```python
from build123d import *

# Parameters (mm, degrees)
AUFSATZ_LINEAR_AUSTRAGEN1_DEPTH = 380


with BuildPart() as part:
    # Skizze1 → Aufsatz-Linear austragen1 (new body)
    with BuildSketch(Plane.XY):
        with BuildLine():
            Line((9.896623228, -8.686160957), (9.896623228, -3.686160957))
            Line((9.896623228, -3.686160957), (9.396623228, -3.686160957))
            Line((9.396623228, -3.686160957), (9.396623228, -3.186160957))
            Line((9.396623228, -3.186160957), (8.396623228, -3.186160957))
            Line((8.396623228, -3.186160957), (8.396623228, -6.186160957))
            Line((8.396623228, -6.186160957), (6.957283398, -6.186160957))
            Line((6.957283398, -6.186160957), (4.396623228, -3.625500787))
            Line((4.396623228, -3.625500787), (4.396623228, 3.253178873))
            Line((4.396623228, 3.253178873), (6.957283398, 5.813839043))
            Line((6.957283398, 5.813839043), (8.396623228, 5.813839043))
            Line((8.396623228, 5.813839043), (8.396623228, 2.813839043))
            Line((8.396623228, 2.813839043), (9.396623228, 2.813839043))
            Line((9.396623228, 2.813839043), (9.396623228, 3.313839043))
            Line((9.396623228, 3.313839043), (9.896623228, 3.313839043))
            Line((9.896623228, 3.313839043), (9.896623228, 8.313839043))
            ThreePointArc((9.896623228, 8.313839043), (9.457283398, 9.374499213), (8.396623228, 9.813839043))
            Line((8.396623228, 9.813839043), (3.396623228, 9.813839043))
            Line((3.396623228, 9.813839043), (3.396623228, 9.313839043))
            Line((3.396623228, 9.313839043), (2.896623228, 9.313839043))
            Line((2.896623228, 9.313839043), (2.896623228, 8.313839043))
            Line((2.896623228, 8.313839043), (5.896623228, 8.313839043))
            Line((5.896623228, 8.313839043), (5.896623228, 6.874499213))
            Line((5.896623228, 6.874499213), (3.335963058, 4.313839043))
            Line((3.335963058, 4.313839043), (-3.542716602, 4.313839043))
            Line((-3.542716602, 4.313839043), (-6.103376772, 6.874499213))
            Line((-6.103376772, 6.874499213), (-6.103376772, 8.313839043))
            Line((-6.103376772, 8.313839043), (-3.103376772, 8.313839043))
            Line((-3.103376772, 8.313839043), (-3.103376772, 9.313839043))
            Line((-3.103376772, 9.313839043), (-3.603376772, 9.313839043))
            Line((-3.603376772, 9.313839043), (-3.603376772, 9.813839043))
            Line((-3.603376772, 9.813839043), (-8.603376772, 9.813839043))
            ThreePointArc((-8.603376772, 9.813839043), (-9.664036942, 9.374499213), (-10.103376772, 8.313839043))
            Line((-10.103376772, 8.313839043), (-10.103376772, 3.313839043))
            Line((-10.103376772, 3.313839043), (-9.603376772, 3.313839043))
            Line((-9.603376772, 3.313839043), (-9.603376772, 2.813839043))
            Line((-9.603376772, 2.813839043), (-8.603376772, 2.813839043))
            Line((-8.603376772, 2.813839043), (-8.603376772, 5.813839043))
            Line((-8.603376772, 5.813839043), (-7.164036942, 5.813839043))
            Line((-7.164036942, 5.813839043), (-4.603376772, 3.253178873))
            Line((-4.603376772, 3.253178873), (-4.603376772, -3.625500787))
            Line((-4.603376772, -3.625500787), (-7.164036942, -6.186160957))
            Line((-7.164036942, -6.186160957), (-8.603376772, -6.186160957))
            Line((-8.603376772, -6.186160957), (-8.603376772, -3.186160957))
            Line((-8.603376772, -3.186160957), (-9.603376772, -3.186160957))
            Line((-9.603376772, -3.186160957), (-9.603376772, -3.686160957))
            Line((-9.603376772, -3.686160957), (-10.103376772, -3.686160957))
            Line((-10.103376772, -3.686160957), (-10.103376772, -8.686160957))
            ThreePointArc((-10.103376772, -8.686160957), (-9.664036942, -9.746821127), (-8.603376772, -10.186160957))
            Line((-8.603376772, -10.186160957), (-3.603376772, -10.186160957))
            Line((-3.603376772, -10.186160957), (-3.603376772, -9.686160957))
            Line((-3.603376772, -9.686160957), (-3.103376772, -9.686160957))
            Line((-3.103376772, -9.686160957), (-3.103376772, -8.686160957))
            Line((-3.103376772, -8.686160957), (-6.103376772, -8.686160957))
            Line((-6.103376772, -8.686160957), (-6.103376772, -7.246821127))
            Line((-6.103376772, -7.246821127), (-3.542716602, -4.686160957))
            Line((-3.542716602, -4.686160957), (3.335963058, -4.686160957))
            Line((3.335963058, -4.686160957), (5.896623228, -7.246821127))
            Line((5.896623228, -7.246821127), (5.896623228, -8.686160957))
            Line((5.896623228, -8.686160957), (2.896623228, -8.686160957))
            Line((2.896623228, -8.686160957), (2.896623228, -9.686160957))
            Line((2.896623228, -9.686160957), (3.396623228, -9.686160957))
            Line((3.396623228, -9.686160957), (3.396623228, -10.186160957))
            Line((3.396623228, -10.186160957), (8.396623228, -10.186160957))
            ThreePointArc((8.396623228, -10.186160957), (9.457283398, -9.746821127), (9.896623228, -8.686160957))
        make_face()
        with BuildLine():
            Line((-2.539013132, 1.090622313), (-3.103550972, 1.763412313))
            Line((-3.103550972, 1.763412313), (-2.052950042, 2.814013243))
            Line((-2.052950042, 2.814013243), (-1.380160042, 2.249475403))
            ThreePointArc((-1.380160042, 2.249475403), (-0.103376772, 2.563839041), (1.173406498, 2.249475399))
            Line((1.173406498, 2.249475399), (1.846196498, 2.814013239))
            Line((1.846196498, 2.814013239), (2.896797428, 1.763412309))
            Line((2.896797428, 1.763412309), (2.332259586, 1.09062231))
            ThreePointArc((2.332259586, 1.09062231), (2.646623225, -0.186160958), (2.332259587, -1.462944226))
            Line((2.332259587, -1.462944226), (2.896797427, -2.135734226))
            Line((2.896797427, -2.135734226), (1.846196497, -3.186335156))
            Line((1.846196497, -3.186335156), (1.173406497, -2.621797316))
            ThreePointArc((1.173406497, -2.621797316), (-0.103376773, -2.936160957), (-1.380160043, -2.62179732))
            Line((-1.380160043, -2.62179732), (-2.052950043, -3.18633516))
            Line((-2.052950043, -3.18633516), (-3.103550973, -2.13573423))
            Line((-3.103550973, -2.13573423), (-2.539013133, -1.46294423))
            ThreePointArc((-2.539013133, -1.46294423), (-2.853376773, -0.186160958), (-2.539013132, 1.090622313))
        make_face(mode=Mode.SUBTRACT)
    extrude(amount=AUFSATZ_LINEAR_AUSTRAGEN1_DEPTH)


solid = part.part
```
Check sheet for the modelled part. Datum: model origin and axes. Units: mm. Round coordinates to 2 decimals unless told otherwise and drop trailing zeros. Write item = value, one per line. Start each with the question number.
1) Thickness scan on probe 1 along X at (y, z) = (-3.5, 61); probe 2 along X at (y, z) = (0, 363); probe 3 along X at (y, z) = (-2, 340.5). Record the ranges inside material, lowest first.
2) Release check for a two-part mould opening along Y. For faces 1 (the flat face through (-4.603, 0, 187)), 2 (the flat face through (4, 0, 380)) record: released by +Y, released by -Y, zero draft, split by the parting line, or undercut.
3) Gauge pin test, flat ends, axial feed: pin 1 Ø8 at (x, y) = (-7, 7.5) entering from -Z; pin 2 Ø4 at (x, z) = (-1, 248.5) entering from +Y; pin 3 Ø0.6 at (y, z) = (9.5, 163) entering from -X; pin 4 Ø0.6 at (y, z) = (-10, 101.5) entering from -X. Record the tip position at first contact, or that the pin passes through.
Results are:
q1.probe_1 = -9.6 to -8.6, -4.6 to 4.4, 8.4 to 9.4
q1.probe_2 = -4.6 to -2.85, 2.64 to 4.4
q1.probe_3 = -4.6 to -2.99, 2.78 to 4.4
q2.face_1 = undercut
q2.face_2 = zero draft
q3.pin_1 = 0
q3.pin_2 = 4.31
q3.pin_3 = -9.81
q3.pin_4 = -9.71
